Could you check a few things on this model? Use its own coordinates, in mm. Coordinates: 2 decimals unless noted, no trailing zeros. Write each loop counter-clockwise with the first axis right and the second up, starting at its lowest first coordinate (ties: lowest second). Pieces come first, ordered by that corner, then holes. Notation, with made-up numbers: M 29.25,51 L 59.25,51 A19 cw 59.25,88 Z; hole C 73.5,38 d1. An arc over 180 degrees is marked long. Answer as CSV lines item,"result". Start each with the question number.
Item 1: Suppose I cut it at B-B, the plane y = -26. Write out the boundary of the cut face in (x, z).
Item 2: Suppose I cut it at D-D, the plane y = 2.5. Write out the boundary of the cut face in (x, z), and give its area (3 significant figures).
Item 3: Suppose I cut it at C-C, the plane x = -6. Write out the boundary of the cut face in (y, z), and give its area (3 significant figures).
Item 4: If I drill on line 1 along Z through (x, y) = (3.5, -3); line 2 along Y through (x, z) = (-3.5, 0.5); line 3 along X through (y, z) = (22, 6), over which ranges is the centre line in solid material (lowest first)? Write a range as [from, to].
Item 5: I'm going to push flat-ended pins straight in: P1, Ø6.5, axis at x = -0.1, y = -26, coming from the +Z side; P2, Ø1.8, axis at y = 22.5, z = 4, coming from the +X side; P3, Ø4, axis at x = -11.5, y = 23.5, coming from the +Z side; P4, Ø2.5, axis at x = 0.5, z = 5.5, coming from the -Y side. Where does each tip first touch, or does it pass through?
Item 6: Suppose I cut it at A-A, the plane z = 0.75. Write out the boundary of the cut face in (x, y), and give its area (3 significant figures).
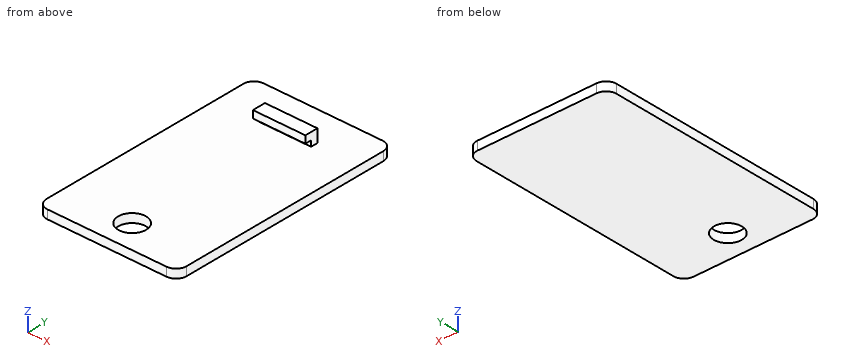
```python
from build123d import *

# Parameters (mm, degrees)
F0_W     = 40
F0_H     = 68
F0_R     = 4
F1_DEPTH = 2.5
F2_R     = 3
F3_W     = 15
F3_H     = 3.8
F4_DEPTH = 3.7
F5_W     = 1.8
F5_H     = 1.6
F6_DEPTH = 25


with BuildPart() as f1:
    # F0 (on Top) → F1 (new body)
    with BuildSketch(Plane.XY):
        Rectangle(F0_W, F0_H)
        with Locations((-0.09511, -26)):
            Circle(F0_R, mode=Mode.SUBTRACT)
    extrude(amount=F1_DEPTH)

    # F2
    f2_edges = [f1.edges().sort_by_distance(p)[0] for p in [
        (-20, 34, 1.25),
        (20, 34, 1.25),
        (-20, -34, 1.25),
        (20, -34, 1.25),
    ]]
    fillet(f2_edges, radius=F2_R)

    # F3 (on face) → F4 (join)
    with BuildSketch(Plane.XY.offset(2.5)):
        with Locations((0, 22.1)):
            Rectangle(F3_W, F3_H)
    extrude(amount=F4_DEPTH)

    # F5 (on face) → F6 (cut)
    with BuildSketch(Plane(origin=(-7.5, 0, 0), x_dir=(0, -1, 0), z_dir=(-1, 0, 0))):
        with Locations((-21.1, 3.3)):
            Rectangle(F5_W, F5_H)
    extrude(amount=-F6_DEPTH, mode=Mode.SUBTRACT)


solid = f1.part
```
Ans:
1,outline,"M -20,0 L -4.1,0 L -4.1,2.5 L -20,2.5 Z; M 3.9,0 L 20,0 L 20,2.5 L 3.9,2.5 Z"
2,outline,"M -20,0 L 20,0 L 20,2.5 L -20,2.5 Z"
2,area,"100 mm^2"
3,outline,"M -34,0 L 34,0 L 34,2.5 L 24,2.5 L 24,6.2 L 20.2,6.2 L 20.2,4.1 L 22,4.1 L 22,2.5 L -34,2.5 Z"
3,area,"181 mm^2"
4,line 1,"z = [0, 2.5]"
4,line 2,"y = [-34, -28.1], [-23.9, 34]"
4,line 3,"x = [-7.5, 7.5]"
5,P1,"passes through"
5,P2,"stops at x = 7.5"
5,P3,"stops at z = 2.5"
5,P4,"stops at y = 20.2"
6,outline,"M -20,-31 A3 ccw -17,-34 L 17,-34 A3 ccw 20,-31 L 20,31 A3 ccw 17,34 L -17,34 A3 ccw -20,31 Z; hole C -0.1,-26 d8"
6,area,"2,660 mm^2"
